Build history of the part. All positions in model axes, mm. Face numbers are marked on the shaded views. A direction names the side the tool comes from. Round coordinates to 2 decimals unless told otherwise and drop trailing zeros. Write each loop counter-clockwise with the first axis right and the second up, starting at its lowest first coordinate (ties: lowest second). Pieces come first, ordered by that corner, then holes.
Item 1: Band-saw the part on A-A, the plane x = 0. Write the cut outline in (y, z).
Item 2: Drop flat-ended pins along their axis: pin 1 Ø1.5 at (x, z) = (-16, 25) entering from -Y; pin 2 Ø2 at (x, z) = (3, 14.5) entering from +Y; pin 3 Ø12 at (x, z) = (-7, 3.5) entering from +Y; pin 4 Ø1.5 at (x, y) = (6, -16.5) entering from +Z. Give the stop position or say it passes through.
Item 3: 3-axis set-ups, long thin cutter, end or side, ignore diameter. For the marked faces 4 and 5: which of +Z, -Z, +X, -X, +Y, -Y reach the whole face in a straight line?
Item 4: Band-saw the part on D-D, the plane y = 8.5. Write the cut outline in (x, z).
Item 5: Wall check: probe 1 along Y at (x, z) = (0, 20.5); probe 2 along X at (y, z) = (-87, 14.75); probe 3 along Z at (x, y) = (7, -27). Give the ranges that are in metal, low to high.
Item 6: Mould opens along X. For the marked faces 1, 2 and 3 say: +X half, -X half, draft (parallel to the pull), parting line (faces both ways), or undercut.
Item 7: Band-saw the part on C-C, the plane y = -60. Write the cut outline in (x, z), then the cut area to 3 significant figures.
Item 8: Band-saw the part on B-B, the plane z = 23.25. Write the cut outline in (x, y).
```python
from build123d import *

# Parameters (mm, degrees)
SKETCH1_R           = 22
SKETCH1_R_2         = 19
BOSS_EXTRUDE1_DEPTH = 30
SKETCH2_W           = 40
SKETCH2_H           = 70
CUT_EXTRUDE1_DEPTH  = 25
SKETCH3_W           = 44
SKETCH3_H           = 13
CUT_EXTRUDE2_DEPTH  = 117.120626936
SKETCH4_W           = 40
SKETCH4_H           = 25
CUT_EXTRUDE3_DEPTH  = 25


with BuildPart() as part:
    # Sketch1 → Boss-Extrude1 (new body)
    # profile 1 of 2: a face of its own
    with BuildSketch(Plane.XY):
        Circle(SKETCH1_R)
        Circle(SKETCH1_R_2, mode=Mode.SUBTRACT)
    # profile 2 of 2: a face of its own
    with BuildSketch(Plane.XY):
        with BuildLine():
            Line((22, -110), (22, 0))
            ThreePointArc((22, 0), (0, -22), (-22, 0))
            Line((-22, 0), (-22, -110))
            Line((-22, -110), (22, -110))
        make_face()
    extrude(amount=BOSS_EXTRUDE1_DEPTH)

    # Sketch2 → Cut-Extrude1 (cut)
    with BuildSketch(Plane.XY.offset(30)):
        with Locations((0, -60)):
            Rectangle(SKETCH2_W, SKETCH2_H)
    extrude(amount=-CUT_EXTRUDE1_DEPTH, mode=Mode.SUBTRACT)

    # Sketch3 → Cut-Extrude2 (cut, through all)
    with BuildSketch(Plane.XY.offset(30)):
        with Locations((0, -103.5)):
            Rectangle(SKETCH3_W, SKETCH3_H)
    extrude(amount=-CUT_EXTRUDE2_DEPTH, mode=Mode.SUBTRACT)

    # Sketch4 → Cut-Extrude3 (cut)
    with BuildSketch(Plane(origin=(0, -95, 0), x_dir=(1, 0, 0), z_dir=(0, 1, 0))):
        with Locations((0, -17.5)):
            Rectangle(SKETCH4_W, SKETCH4_H)
    extrude(amount=-CUT_EXTRUDE3_DEPTH, mode=Mode.SUBTRACT)


solid = part.part
```
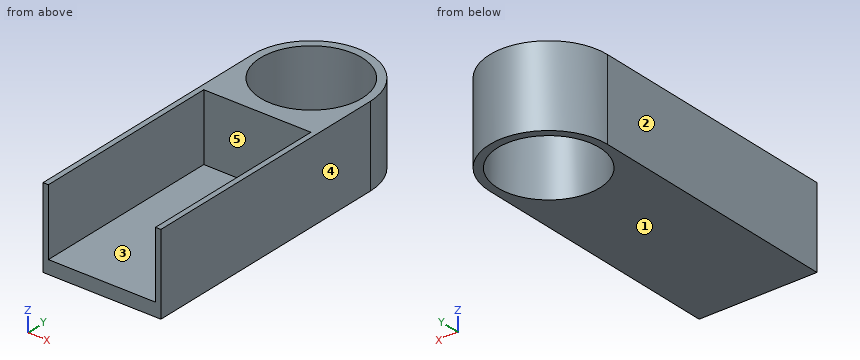
Results:
1. outline: (-97, 0) - (-19, 0) - (-19, 30) - (-25, 30) - (-25, 5) - (-97, 5) - close; (19, 0) - (22, 0) - (22, 30) - (19, 30) - close
2. pin 1: stops at y = -25
2. pin 2: stops at y = 21.91
2. pin 3: stops at y = 21.98
2. pin 4: passes through
3. face 4: +Z, -Z, +X, +Y, -Y
3. face 5: +Z, -Y
4. outline: (-20.29, 0) - (-16.99, 0) - (-16.99, 30) - (-20.29, 30) - close; (16.99, 0) - (20.29, 0) - (20.29, 30) - (16.99, 30) - close
5. probe 1: y = -25 to -19, 19 to 22
5. probe 2: x = -22 to -20, 20 to 22
5. probe 3: z = 0 to 5
6. face 1: draft
6. face 2: -X half
6. face 3: undercut
7. outline: (-22, 0) - (22, 0) - (22, 30) - (20, 30) - (20, 5) - (-20, 5) - (-20, 30) - (-22, 30) - close
7. area: 320 mm2
8. outline: (-22, -97) - (-20, -97) - (-20, -25) - (20, -25) - (20, -97) - (22, -97) - (22, 0) arc R22 ccw to (-22, 0) - close; hole circle Ø38 at (0, 0)
